```python
from build123d import *

# Parameters (mm, degrees)
F0_W      = 5.842
F0_H      = 12.7
F0_R      = 3.175
F2_DEPTH  = 3.175
F3_R      = 1.524
F4_DEPTH  = 6.35
F5_DEPTH  = 1.27
F6_DEPTH  = 6.35
F7_DEPTH  = 56.134
F8_R      = 1.524
F9_DEPTH  = 10.414
F10_R     = 1.524
F11_DEPTH = 17.78


with BuildPart() as f1:
    # F0 (on Front) → F1 (revolve)
    with BuildSketch(Plane.XZ):
        Polygon((5.842, 12.7), (5.842, 0), (66.294, 0), (66.294, 12.7), (56.134, 12.7), (56.134, 10.16), (10.16, 10.16), (10.16, 12.7), align=None)
        with Locations((2.921, 6.35)):
            Rectangle(F0_W, F0_H)
    revolve(axis=Axis((33.147, 0, 0), (-1, 0, 0)))

    # F0 (on Front) → F2 (join, symmetric)
    with BuildSketch(Plane.XZ):
        with Locations((2.921, 6.35)):
            Rectangle(F0_W, F0_H)
        with BuildLine():
            Line((-0.9398, 0), (0, 0))
            Line((0, 0), (0, 12.7))
            Line((0, 12.7), (5.842, 12.7))
            Line((5.842, 12.7), (5.842, 15.24))
            Line((5.842, 15.24), (-0.508, 15.24))
            Line((-0.508, 15.24), (-10.8806298187, 3.8475430269))
            ThreePointArc((-10.8806298187, 3.8475430269), (-4.5919612295, 5.3297205562), (-0.9398, 0))
        make_face()
        with BuildLine():
            Line((5.842, 0), (0, 0))
            Line((0, 0), (-0.9398, 0))
            ThreePointArc((-0.9398, 0), (-3.1957909266, -4.5493385486), (-8.1826630726, -5.5069827884))
            Line((-8.1826630726, -5.5069827884), (5.842, -9.398))
            Line((5.842, -9.398), (5.842, 0))
        make_face()
        with BuildLine():
            ThreePointArc((-8.1826630726, -5.5069827884), (-3.1957909266, -4.5493385486), (-0.9398, 0))
            ThreePointArc((-0.9398, 0), (-4.5919612295, 5.3297205562), (-10.8806298187, 3.8475430269))
            ThreePointArc((-10.8806298187, 3.8475430269), (-12.1459778134, -1.5837270034), (-8.1826630726, -5.5069827884))
        make_face()
        with Locations((-6.6548, 0)):
            Circle(F0_R, mode=Mode.SUBTRACT)
    extrude(amount=F2_DEPTH, both=True)

    # F3 (on face) → F4 (join)
    with BuildSketch(Plane.YZ.offset(66.294)):
        with BuildLine():
            ThreePointArc((-5.08, 0), (0, 5.08), (5.08, 0))
            Line((5.08, 0), (5.08, 11.6397422652))
            ThreePointArc((5.08, 11.6397422652), (0, 12.7), (-5.08, 11.6397422652))
            Line((-5.08, 11.6397422652), (-5.08, 0))
        make_face()
        with BuildLine():
            ThreePointArc((-5.08, 0), (0, -5.08), (5.08, 0))
            ThreePointArc((5.08, 0), (0, 5.08), (-5.08, 0))
        make_face()
        Circle(F3_R, mode=Mode.SUBTRACT)
        with BuildLine():
            ThreePointArc((-5.08, 11.6397422652), (0, 12.7), (5.08, 11.6397422652))
            Line((5.08, 11.6397422652), (5.08, 15.24))
            Line((5.08, 15.24), (3.175, 15.24))
            Line((3.175, 15.24), (-3.175, 15.24))
            Line((-3.175, 15.24), (-5.08, 15.24))
            Line((-5.08, 15.24), (-5.08, 11.6397422652))
        make_face()
        Circle(F3_R)
    extrude(amount=F4_DEPTH)

    # F3 (on face) → F5 (join)
    with BuildSketch(Plane.YZ.offset(66.294)):
        with BuildLine():
            ThreePointArc((-5.08, 0), (0, -5.08), (5.08, 0))
            ThreePointArc((5.08, 0), (0, 5.08), (-5.08, 0))
        make_face()
        Circle(F3_R, mode=Mode.SUBTRACT)
        with BuildLine():
            ThreePointArc((-5.08, 0), (0, 5.08), (5.08, 0))
            Line((5.08, 0), (5.08, 15.24))
            Line((5.08, 15.24), (3.175, 15.24))
            Line((3.175, 15.24), (-3.175, 15.24))
            Line((-3.175, 15.24), (-5.08, 15.24))
            Line((-5.08, 15.24), (-5.08, 0))
        make_face()
    extrude(amount=-F5_DEPTH)

    # F3 (on face) → F6 (cut)
    with BuildSketch(Plane.YZ.offset(66.294)):
        Circle(F3_R)
    extrude(amount=F6_DEPTH, mode=Mode.SUBTRACT)

    # F3 (on face) → F7 (cut, through all)
    with BuildSketch(Plane.YZ.offset(66.294)):
        Circle(F3_R)
    extrude(amount=-F7_DEPTH, mode=Mode.SUBTRACT)

    # F8 (on face) → F9 (cut)
    with BuildSketch(Plane.XY.offset(15.24)):
        with Locations((68.834, 0)):
            Circle(F8_R)
    extrude(amount=-F9_DEPTH, mode=Mode.SUBTRACT)

    # F10 (on face) → F11 (cut)
    with BuildSketch(Plane.XY.offset(15.24)):
        with Locations((2.667, 0)):
            Circle(F10_R)
    extrude(amount=-F11_DEPTH, mode=Mode.SUBTRACT)


solid = f1.part
```
Check sheet for the modelled part. Datum: model origin and axes. Units: mm. A direction names the side the tool comes from. Give positions to 0.01 mm unless a question says otherwise; leave off trailing zeros. Order: outer loops, then holes, each group sorted by start corner. A loop starts at its lowest first (then second) coordinate and runs counter-clockwise, first axis right, second up. Notation, with made-up numbers: M -20.75,23.25 L -10.75,23.25 A27 cw -10.75,58.25 Z; hole C -11.5,6 d1. An arc over 180 degrees is marked long. Answer in a Markdown table with one row per item. Add a question column.
Q1. Sectioned sample at A-A, the plane x = -6.5. Record the boundary of the cut face in (y, z) (3 decimals), and give its area (3 significant figures).
Q2. Release check for a two-part mould opening along X. For faces 5 (the flat face through (10.16, 9, 6)), 6 (the flat face through (72.644, 0, 5)), 7 (the cylindrical face through (-3.626, 0.044, 0.954)), 8 (the flat face through (71, 0, 15.24)) record: released by +X, released by -X, zero draft, split by the parting line, or undercut.
Q3. Access from +Z, -Z, +X, -X, +Y, -Y to the whole of each face (thin tool, end or side, straight path). Record for faces 1 (the flat face through (3, 0, -2.54)), 2 (the flat face through (56.134, 9, -6)), 3 (the cylindrical face through (69.42, -0.11, -5.08)), 4 (the cylindrical face through (40.96, -0.2, 1.51)).
Q4. Sectioned sample at D-D, the plane x = 47. Record the boundary of the cut face in (y, z), and give its area (3 significant figures).
Q5. Gauge pin test, flat ends, axial feed: pin 1 Ø6 at (y, z) = (-8.5, 2.5) entering from -X; pin 2 Ø12 at (x, z) = (62.5, -8) entering from -Y; pin 3 Ø3.5 at (x, y) = (69.5, -0.5) entering from +Z; pin 4 Ø5.5 at (x, z) = (-7.5, 1.5) entering from +Y (3 decimals). Record the tip position at first contact, or that the pin passes through.
Q6. Thickness scan on L1, parallel to X at y = -8, z = -9.75; L2, parallel to X at y = -3.5, z = 7.75; L3, parallel to Z at x = 2.5, y = 0.25. Record the ranges inside material, lowest first.
Q7. Sectioned sample at B-B, the plane z = 13.5. Record the boundary of the cut face in (x, y) (3 decimals), and give its area (3 significant figures).
Verdict:
| question | item | result |
|---|---|---|
| 1 | outline | M -3.175,-5.974 L 3.175,-5.974 L 3.175,-3.171 L -3.175,-3.171 Z; M -3.175,3.171 L 3.175,3.171 L 3.175,8.659 L -3.175,8.659 Z |
| 1 | area | 52.6 mm² |
| 2 | face 5 | undercut |
| 2 | face 6 | released by +X |
| 2 | face 7 | undercut |
| 2 | face 8 | zero draft |
| 3 | face 1 | +Z |
| 3 | face 2 | none |
| 3 | face 3 | -Z, +X |
| 3 | face 4 | +X |
| 4 | outline | C 0,0 d20.32; hole C 0,0 d3.05 |
| 4 | area | 317 mm² |
| 5 | pin 1 | x = 0 |
| 5 | pin 2 | y = -12.54 |
| 5 | pin 3 | z = 15.24 |
| 5 | pin 4 | y = 3.175 |
| 6 | L1 | 0 to 10.16, 56.13 to 66.29 |
| 6 | L2 | 0 to 72.64 |
| 6 | L3 | -12.7 to -2.54 |
| 7 | outline | M -2.092,-3.175 L 5.842,-3.175 L 5.842,3.175 L -2.092,3.175 Z; M 65.024,-5.08 L 72.644,-5.08 L 72.644,5.08 L 65.024,5.08 Z; hole C 2.667,0 d3.048; hole C 68.834,0 d3.048 |
| 7 | area | 113 mm² |
